Input: dimensioned drawing with shaded views. Units: mm. Origin: part minimum x, y, z. Coordinates: 2 decimals unless noted, no trailing zeros. Order: outer loops, then holes, each group sorted by start corner. A loop starts at its lowest first (then second) coordinate and runs counter-clockwise, first axis right, second up. Notation, with made-up numbers: (-28.75, -31.5) -> (4.25, -31.5) arc R10 cw to (4.25, -26.5) -> close; hole circle Ø2 at (-25, 41). An arc over 180 degrees is marked (long way). Write item = value, one per line. Start each with the question number.
Item 1: Section query A-A (x = 8). Output: boundary loops of the cut face in (y, z).
Item 2: Mould query, pull axis Z, two halves, no side actions, for the marked faces 1, 2 and 3. Classes: released by +Z, released by -Z, zero draft, split by the parting line, or undercut.
Item 3: Ray query, line 1 along X through (y, z) = (3.5, 8); line 2 along Y through (x, z) = (1, 5); line 3 along X through (y, z) = (1, 10). Return the intervals inside material, ascending. Write a range as [from, to].
Item 4: Section query B-B (z = 8). Output: boundary loops of the cut face in (x, y), then the cut area to 3 significant figures.
Item 5: Section query C-C (y = 7.25). Output: boundary loops of the cut face in (x, z).
Item 6: Contact query for flat-ended pins moving along their axis: pin 1 (1 mm diameter, centred on x = 5, y = 6.5, fed in from +Z); pin 2 (3 mm diameter, centred on y = 4, z = 3, fed in from +X); pin 3 (2 mm diameter, centred on y = 2, z = 10, fed in from -X). Output: stop coordinate, or through.
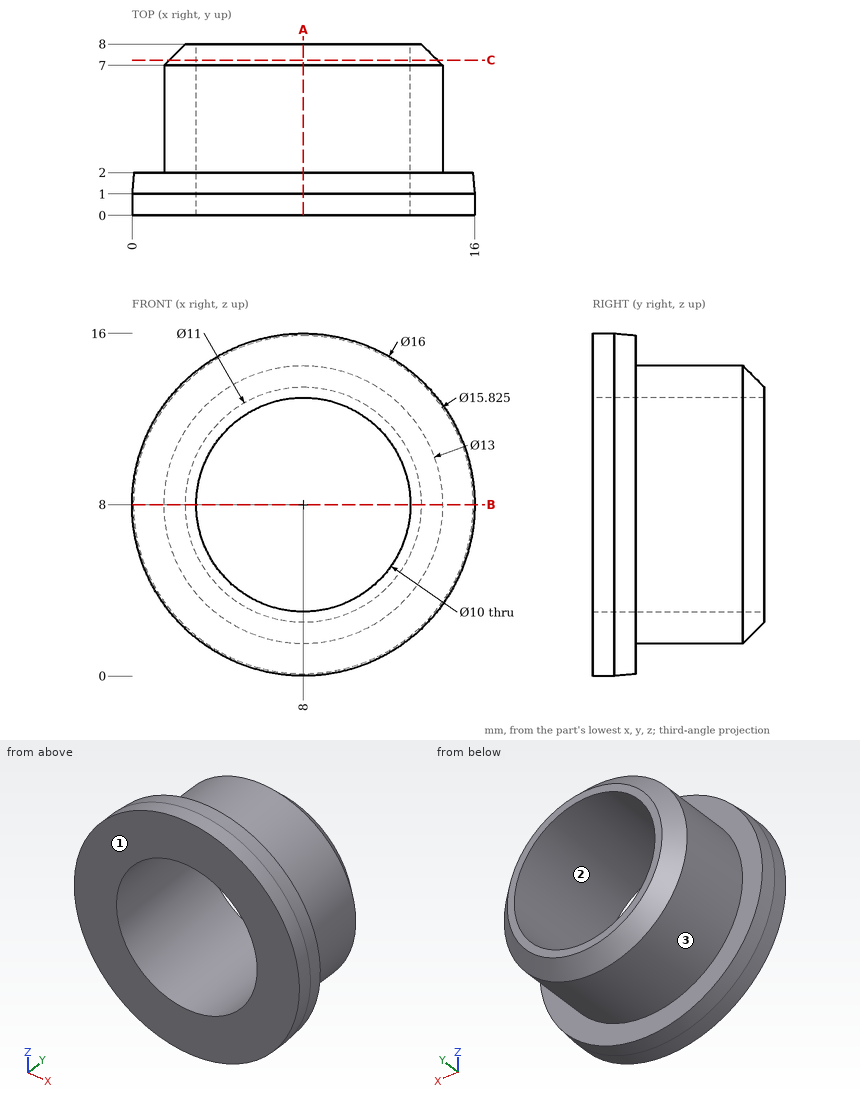
Computed:
q1.outline = (0, 0) -> (1, 0) -> (2, 0.09) -> (2, 1.5) -> (7, 1.5) -> (8, 2.5) -> (8, 3) -> (0, 3) -> close; (0, 13) -> (8, 13) -> (8, 13.5) -> (7, 14.5) -> (2, 14.5) -> (2, 15.91) -> (1, 16) -> (0, 16) -> close
q2.face_1 = zero draft
q2.face_2 = undercut
q2.face_3 = split by the parting line
q3.line_1 = [1.5, 3], [13, 14.5]
q3.line_2 = [0, 2]
q3.line_3 = [0.25, 3.42], [12.58, 15.75]
q4.outline = (0, 0) -> (3, 0) -> (3, 8) -> (2.5, 8) -> (1.5, 7) -> (1.5, 2) -> (0.09, 2) -> (0, 1) -> close; (13, 0) -> (16, 0) -> (16, 1) -> (15.91, 2) -> (14.5, 2) -> (14.5, 7) -> (13.5, 8) -> (13, 8) -> close
q4.area = 28.9 mm^2
q5.outline = circle Ø12.5 at (8, 8); hole circle Ø10 at (8, 8)
q6.pin_1 = 14
q6.pin_2 = 13.48
q6.pin_3 = 0.12
